```python
from build123d import *

# Parameters (mm, degrees)
EXTRUDE_1_DEPTH     = 4
SKETCH_1_W          = 10
SKETCH_1_H          = 10
EXTRUDE_2_DEPTH     = 30
SKETCH_6_W          = 10
SKETCH_6_H          = 10
EXTRUDE_4_DEPTH     = 30
SKETCH_9_R          = 7
SKETCH_9_R_2        = 6
EXTRUDE_5_DEPTH     = 4
SKETCH_11_R         = 4
CUT_EXTRUDE_1_DEPTH = 30


with BuildPart() as part:
    # 草图2 → 凸台-拉伸1 (new body)
    with BuildSketch(Plane(origin=(0, 0, 0), x_dir=(1, 0, 0), z_dir=(0, 1, 0))):
        Polygon((-5, -22), (5, -22), (5, -12), (15, -5), (25, -5), (25, 5), (-25, 5), (-25, -5), (-15, -5), (-5, -12), align=None)
    extrude(amount=EXTRUDE_1_DEPTH)

    # 草图1 → 凸台-拉伸2 (add)
    with BuildSketch(Plane(origin=(0, 0, 0), x_dir=(1, 0, 0), z_dir=(0, 1, 0))):
        with Locations((-20, 0)):
            Rectangle(SKETCH_1_W, SKETCH_1_H)
        with Locations((20, 0)):
            Rectangle(SKETCH_1_W, SKETCH_1_H)
    extrude(amount=-EXTRUDE_2_DEPTH)

    # 草图6 → 凸台-拉伸4 (add)
    with BuildSketch(Plane.XZ):
        with Locations((0, 17)):
            Rectangle(SKETCH_6_W, SKETCH_6_H)
    extrude(amount=EXTRUDE_4_DEPTH)

    # 草图9 → 凸台-拉伸5 (add)
    with BuildSketch(Plane(origin=(0, 4, 0), x_dir=(1, 0, 0), z_dir=(0, 1, 0))):
        with Locations((0, -3.6)):
            Circle(SKETCH_9_R)
        with Locations((0, -3.6)):
            Circle(SKETCH_9_R_2, mode=Mode.SUBTRACT)
    extrude(amount=EXTRUDE_5_DEPTH)

    # 草图11 → 切除-拉伸1 (cut)
    with BuildSketch(Plane.XZ.offset(30)):
        with Locations((0, 17)):
            Circle(SKETCH_11_R)
        with Locations((20, 0)):
            Circle(SKETCH_11_R)
        with Locations((-20, 0)):
            Circle(SKETCH_11_R)
    extrude(amount=-CUT_EXTRUDE_1_DEPTH, mode=Mode.SUBTRACT)


solid = part.part
```
Input: part model. Units: mm. Frame: model coordinates. A direction names the side the tool comes from. Give positions to 0.01 mm unless a question says otherwise; leave off trailing zeros. Loops run counter-clockwise (first coordinate to the right, second up) from the corner with the lowest first, then second, coordinate; pieces in that order, holes last. Notation, with made-up numbers: (-31, 85.5) -> (-14, 85.5) arc R14 ccw to (-14, 99.5) -> close; hole circle Ø10 at (14, -34.75). An arc over 180 degrees is marked (long way). Use a Markdown table: item, result.
Q1. First-contact query: P1, Ø4, axis at x = -8.5, y = -24, coming from the +Z side; P2, Ø12, axis at x = 4, y = -22.5, coming from the -Z side; P3, Ø4, axis at x = 19.5, z = 1, coming from the -Y side; P4, Ø11, axis at y = -5, z = 16.5, coming from the -X side. Flat tips, straight axial feed; report the tip coordinate or a pass-through.
Entries:
| item | result |
|---|---|
| P1 | passes through |
| P2 | stops at z = 12 |
| P3 | stops at y = 0 |
| P4 | stops at x = -5 |
Q2. Section query C-C, the plane z = 7.75. Return the cut outline in (x, y), plus the area to 3 significant figures.
Entries:
| item | result |
|---|---|
| outline | (-11.07, 0) -> (11.07, 0) -> (11.07, 4) -> (5.64, 4) -> (5.64, 8) -> (4.33, 8) -> (4.33, 4) -> (-4.33, 4) -> (-4.33, 8) -> (-5.64, 8) -> (-5.64, 4) -> (-11.07, 4) -> close |
| area | 99.0 mm² |
Q3. Ray query, probe 1 along Z at (x, y) = (-20, -21.25); probe 2 along Z at (x, y) = (0, -22.75); probe 3 along Y at (x, z) = (10, -2.5). Return the intervals inside material, ascending. Write a range as from..to.
Entries:
| item | result |
|---|---|
| probe 1 | z = -5..-4, 4..5 |
| probe 2 | z = 12..13, 21..22 |
| probe 3 | y = 0..4 |
Q4. Pull-direction query (Z, two-part tool) for faces 4 (the flat face through (-25, -13, 0)), 5 (the flat face through (9.93, 1.97, 8.55)), 6 (the cylindrical face through (-4.42, 5.97, -0.46)); classes: pulls with the +Z half, pulls with the -Z half, needs draft (parallel to the pull), parting line crosses it, or undercut.
Entries:
| item | result |
|---|---|
| face 4 | needs draft |
| face 5 | pulls with the +Z half |
| face 6 | undercut |
Q5. Section query A-A, the plane y = -9.5. Return the cut outline in (x, z).
Entries:
| item | result |
|---|---|
| outline | (-25, -5) -> (-15, -5) -> (-15, 5) -> (-25, 5) -> close; (-5, 12) -> (5, 12) -> (5, 22) -> (-5, 22) -> close; (15, -5) -> (25, -5) -> (25, 5) -> (15, 5) -> close; hole circle Ø8 at (-20, 0); hole circle Ø8 at (0, 17); hole circle Ø8 at (20, 0) |
Q6. Section query D-D, the plane x = -20. Return the cut outline in (y, z), plus the area to 3 significant figures.
Entries:
| item | result |
|---|---|
| outline | (-30, -5) -> (4, -5) -> (4, 5) -> (-30, 5) -> (-30, 4) -> (0, 4) -> (0, -4) -> (-30, -4) -> close |
| area | 100 mm² |
Q7. Access query for faces 1 (the flat face through (15, -15, 0)), 2 (the flat face through (0, 4, 4)), 3 (the flat face through (0, 0, 17)). Directions: +Z, -Z, +X, -X, +Y, -Y. A direction counts if a zero-diameter tool reaches every point of the face in a straight line with its end or side. Return the directions, or none.
Entries:
| item | result |
|---|---|
| face 1 | +Z, -Z, -Y |
| face 2 | +Y |
| face 3 | -Y |
Q8. Section query B-B, the plane x = 0. Return the cut outline in (y, z), plus the area to 3 significant figures.
Entries:
| item | result |
|---|---|
| outline | (-30, 12) -> (0, 12) -> (0, -5) -> (4, -5) -> (4, -3.4) -> (8, -3.4) -> (8, -2.4) -> (4, -2.4) -> (4, 9.6) -> (8, 9.6) -> (8, 10.6) -> (4, 10.6) -> (4, 22) -> (-30, 22) -> (-30, 21) -> (0, 21) -> (0, 13) -> (-30, 13) -> close |
| area | 176 mm² |
